Verification items for the finished model (mm, model axes). Face numbers are marked on the shaded views. A direction names the side the tool comes from. Round coordinates to 2 decimals unless told otherwise and drop trailing zeros. Loops run counter-clockwise (first coordinate to the right, second up) from the corner with the lowest first, then second, coordinate; pieces in that order, holes last. Notation, with made-up numbers: (69.25, 38) -> (112.25, 38) arc R29 cw to (112.25, 66) -> close; hole circle Ø6 at (36.25, 1). An arc over 180 degrees is marked (long way). Use a Markdown table: item, result. Add a question column.
```python
from build123d import *

# Parameters (mm, degrees)
PAD_DEPTH       = 5
PAD001_DEPTH    = 50
POCKET_DEPTH    = 4
SKETCH003_R     = 1.5
POCKET001_DEPTH = 17
SKETCH004_R     = 2.25
HOLE_DEPTH      = 25
SKETCH008_W     = 45
SKETCH008_H     = 30
POCKET002_DEPTH = 4


with BuildPart() as part:
    # Sketch → Pad (new body)
    with BuildSketch(Plane.XY):
        Polygon((0, 0), (-10, 0), (-10, 4), (110, 4), (110, 0), (100, 0), (100, -61), (0, -61), align=None)
    extrude(amount=-PAD_DEPTH)

    # Sketch001 → Pad001 (join)
    with BuildSketch(Plane.XY):
        Polygon((0, 0), (-10, 0), (-10, 4), (4, 4), (4, -13), (45, -13), (45, -17), (4, -17), (4, -57), (96, -57), (96, -17), (86, -17), (86, -13), (96, -13), (96, 4), (110, 4), (110, 0), (100, 0), (100, -61), (0, -61), align=None)
    extrude(amount=PAD001_DEPTH)

    # Sketch002 → Pocket (cut)
    with BuildSketch(Plane.YZ):
        with BuildLine():
            Line((-26, 50), (-17, 50))
            Line((-17, 50), (-17, 35))
            ThreePointArc((-26, 35), (-21.5, 30.5), (-17, 35))
            Line((-26, 50), (-26, 35))
        make_face()
    extrude(amount=POCKET_DEPTH, mode=Mode.SUBTRACT)

    # Sketch003 → Pocket001 (cut)
    with BuildSketch(Plane.XZ):
        with Locations((41, 15)):
            Circle(SKETCH003_R)
        with Locations((41, 5)):
            Circle(SKETCH003_R)
        with Locations((91, 15)):
            Circle(SKETCH003_R)
        with Locations((91, 5)):
            Circle(SKETCH003_R)
    extrude(amount=POCKET001_DEPTH, mode=Mode.SUBTRACT)

    # Sketch004 → Hole (cut)
    with BuildSketch(Plane.XZ):
        with Locations((-5, 40)):
            Circle(SKETCH004_R)
        with Locations((-5, 5)):
            Circle(SKETCH004_R)
        with Locations((105, 40)):
            Circle(SKETCH004_R)
        with Locations((105, 5)):
            Circle(SKETCH004_R)
    extrude(amount=-HOLE_DEPTH, mode=Mode.SUBTRACT)

    # Sketch008 (on Face25 of Hole) → Pocket002 (cut)
    with BuildSketch(Plane(origin=(0, -13, 0), x_dir=(-1, 0, 0), z_dir=(0, 1, 0))):
        with Locations((-26.5, 35)):
            Rectangle(SKETCH008_W, SKETCH008_H)
    extrude(amount=-POCKET002_DEPTH, mode=Mode.SUBTRACT)


solid = part.part
```
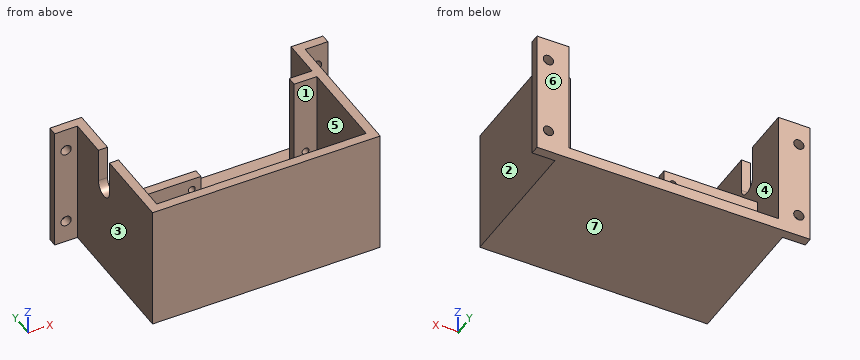
1) Sectioned sample at A-A on z = 15. Enter the section's corners in (x, y), then the cut area to 3 significant figures.
2) Thickness scan on line 1 (X direction, y = -16.05, z = 15); line 2 (Z direction, x = 41, y = -15); line 3 (Z direction, x = 91, y = -14). Record the ranges inside material, lowest first.
3) Sectioned sample at D-D on y = -54. Enter the section's corners in (x, z), then the cut area to 3 significant figures.
4) Sectioned sample at C-C on z = 40. Enter the section's corners in (x, y).
5) Go/stop test with flat-tipped pins: pin 1 (2.5 mm diameter, centred on x = 105, z = 5, fed in from +Y); pin 2 (25 mm diameter, centred on y = -20.5, z = 23, fed in from +X); pin 3 (1.5 mm diameter, centred on x = 45.5, z = 12, fed in from +Y); pin 4 (6 mm diameter, centred on x = 81, z = 24, fed in from +Y). Record where each tip stops, or that it passes through.
6) Release check for a two-part mould opening along Y. For the marked faces 4, 5, 6 and 7 record: released by +Y, released by -Y, zero draft, split by the parting line, or undercut.
7) Sectioned sample at B-B on x = -5. Enter the section's corners in (y, z), then the cut area to 3 significant figures.
8) Access from +Z, -Z, +X, -X, +Y, -Y to the whole of each face (thin tool, end or side, straight path). Record for the marked faces 1, 2 and 3.
Geometry results:
| question | item | result |
|---|---|---|
| 1 | outline | (-10, 0) -> (0, 0) -> (0, -61) -> (100, -61) -> (100, 0) -> (110, 0) -> (110, 4) -> (96, 4) -> (96, -13) -> (92.5, -13) -> (92.5, -17) -> (96, -17) -> (96, -57) -> (4, -57) -> (4, -17) -> (39.5, -17) -> (39.5, -13) -> (4, -13) -> (4, 4) -> (-10, 4) -> close; (42.5, -17) -> (45, -17) -> (45, -13) -> (42.5, -13) -> close; (86, -17) -> (89.5, -17) -> (89.5, -13) -> (86, -13) -> close |
| 1 | area | 1,150 mm^2 |
| 2 | line 1 | 0 to 39.5, 42.5 to 45, 86 to 89.5, 92.5 to 100 |
| 2 | line 2 | -5 to 3.5, 6.5 to 13.5, 16.5 to 20 |
| 2 | line 3 | -5 to 3.5, 6.5 to 13.5, 16.5 to 50 |
| 3 | outline | (0, -5) -> (100, -5) -> (100, 50) -> (96, 50) -> (96, 0) -> (4, 0) -> (4, 50) -> (0, 50) -> close |
| 3 | area | 900 mm^2 |
| 4 | outline | (-10, 0) -> (-7.25, 0) -> (-7.25, 4) -> (-10, 4) -> close; (-2.75, 0) -> (0, 0) -> (0, -17) -> (4, -17) -> (4, 4) -> (-2.75, 4) -> close; (0, -61) -> (100, -61) -> (100, 0) -> (102.75, 0) -> (102.75, 4) -> (96, 4) -> (96, -13) -> (86, -13) -> (86, -17) -> (96, -17) -> (96, -57) -> (4, -57) -> (4, -26) -> (0, -26) -> close; (107.25, 0) -> (110, 0) -> (110, 4) -> (107.25, 4) -> close |
| 5 | pin 1 | through |
| 5 | pin 2 | x = 100 |
| 5 | pin 3 | y = -13 |
| 5 | pin 4 | y = -57 |
| 6 | face 4 | undercut |
| 6 | face 5 | undercut |
| 6 | face 6 | released by +Y |
| 6 | face 7 | zero draft |
| 7 | outline | (0, -5) -> (4, -5) -> (4, 2.75) -> (0, 2.75) -> close; (0, 7.25) -> (4, 7.25) -> (4, 37.75) -> (0, 37.75) -> close; (0, 42.25) -> (4, 42.25) -> (4, 50) -> (0, 50) -> close |
| 7 | area | 184 mm^2 |
| 8 | face 1 | +Z |
| 8 | face 2 | +Z, -Z, +X, -Y |
| 8 | face 3 | +Z, -Z, -X, -Y |
